```python
from build123d import *

# Parameters (mm, degrees)
F0_R     = 33.04
F1_DEPTH = 58
F2_SIZE  = 7.62
F3_T     = -3.81
F4_R     = 2.54
F5_R     = 30.5
F5_R_2   = 29.23
F6_DEPTH = 6.35
F7_R     = 1.26999


# Not quite as in the source:
# - a fillet or chamfer is up to 0.001 mm smaller than in the source, because OpenCascade refuses the exact size


with BuildPart() as f1:
    # F0 (on Top) → F1 (new body)
    with BuildSketch(Plane.XY):
        Circle(F0_R)
    extrude(amount=F1_DEPTH)

    # F2
    f2_edges = [f1.edges().sort_by_distance(p)[0] for p in [
        (-33.04, 0, 0),
    ]]
    chamfer(f2_edges, length=F2_SIZE)

    # F3
    f3_openings = [f1.faces().sort_by_distance(p)[0] for p in [
        (0, 0, 58),
    ]]
    offset(amount=F3_T, openings=f3_openings)

    # F4
    f4_edges = [f1.edges().sort_by_distance(p)[0] for p in [
        (-33.04, 0, 7.62),
        (-25.42, 0, 0),
    ]]
    fillet(f4_edges, radius=F4_R)

    # F5 (on face) → F6 (join)
    with BuildSketch(Plane.XY.offset(58)):
        Circle(F5_R)
        Circle(F5_R_2, mode=Mode.SUBTRACT)
    extrude(amount=F6_DEPTH)

    # F7 (radius 1.27 in the source; OpenCascade refuses exactly that, so slightly less here)
    f7_edges = [f1.edges().sort_by_distance(p)[0] for p in [
        (-30.5, 0, 64.35),
    ]]
    fillet(f7_edges, radius=F7_R)


solid = f1.part
```
Geometry: final body of the model. Coordinates: model frame, mm. A direction names the side the tool comes from. Round coordinates to 2 decimals unless told otherwise and drop trailing zeros. Order: outer loops, then holes, each group sorted by start corner. A loop starts at its lowest first (then second) coordinate and runs counter-clockwise, first axis right, second up. Notation, with made-up numbers: (56.5, 86) -> (77.5, 86) arc R10 ccw to (77.5, 92) -> close; hole circle Ø5 at (-3.75, -39.5). An arc over 180 degrees is marked (long way). Use CSV: the item, a comma, the result in double quotes. Start each with the question number.
1) First-contact query: pin 1 Ø5 at (y, z) = (19.5, 25) entering from +X; pin 2 Ø1.5 at (x, z) = (-10, 20) entering from -Y; pin 3 Ø1.5 at (x, y) = (3.5, -23.5) entering from +Z. Flat tips, straight axial feed; report the tip coordinate or a pass-through.
2) Set-up query: faces 1 (the face through (-5.7, -25.8, 1)), 2 (the face through (0, 0, 3.81)). Return all of +Z, -Z, +X, -X, +Y, -Y with unobstructed straight access to the full face (end or side cutting, diameter ignored); none if empty.
3) Material intervals for line 1 along X through (y, z) = (0, 52); line 2 along X through (y, z) = (-9, 17.5), sorted ascending. Write a range as from..to.
4) Section A-A (z = 28.5). Return the cut outline in (x, y).
5) Draft query along X for faces 3 (the face through (27.88, 8.78, 36.39)), 4 (the face through (0, 0, 0)), 5 (the face through (-24.35, 22.33, 32.99)). Return one class per face: +X half, -X half, draft (parallel to the pull), parting line (faces both ways), or undercut.
Returned:
1,pin 1,"stops at x = 28.33"
1,pin 2,"stops at y = -31.72"
1,pin 3,"stops at z = 4.48"
2,face 1,"-Z"
2,face 2,"+Z"
3,line 1,"x = -33.04..-29.23, 29.23..33.04"
3,line 2,"x = -31.79..-27.81, 27.81..31.79"
4,outline,"circle Ø66.08 at (0, 0); hole circle Ø58.46 at (0, 0)"
5,face 3,"undercut"
5,face 4,"draft"
5,face 5,"parting line"
